Autodesk Inventor part; units mm, degrees
ref_plane "Work Plane1" through (0, -1.5, 0) normal (0, -1, 0) x (1, 0, 0)
ref_plane "YZ Plane" through (0, 0, 0) normal (1, 0, 0) x (0, 1, 0)
ref_plane "XZ Plane" through (0, 0, 0) normal (0, 1, 0) x (-1, 0, 0)
sketch "Sketch2" plane through (0, 0, 0) normal (0, 1, 0) x (-1, 0, 0)
  line L0 (-13.1182, 6.5103) -> (18.7692, 6.5103) construction
  line L1 (18.7692, 6.5103) -> (18.7692, -12.5367) construction
  line L2 (18.7692, -12.5367) -> (-13.1182, -12.5367) construction
  line L3 (-13.1182, -12.5367) -> (-13.1182, 6.5103) construction
  line L4 (-5.4, 3.15) -> (5.4, 3.15)
  line L5 (8.55, 0) -> (8.55, 0)
  line L6 (5.4, -3.15) -> (-5.4, -3.15)
  line L7 (-8.55, 0) -> (-8.55, 0)
  line L8 (-8.55, 3.15) -> (8.55, -3.15) construction
  line L9 (8.55, 3.15) -> (-8.55, -3.15) construction
  arc A0 (8.55, 0) -> (5.4, 3.15) centre (5.4, 0) ccw
  arc A1 (5.4, -3.15) -> (8.55, 0) centre (5.4, 0) ccw
  arc A2 (-5.4, 3.15) -> (-8.55, 0) centre (-5.4, 0) ccw
  arc A3 (-8.55, 0) -> (-5.4, -3.15) centre (-5.4, 0) ccw
  line L10 (5.4, 2.35) -> (-5.4, 2.35)
  line L11 (-7.75, 0) -> (-7.75, 0)
  line L12 (-5.4, -2.35) -> (5.4, -2.35)
  line L13 (7.75, 0) -> (7.75, 0)
  line L14 (7.75, 2.35) -> (-7.75, -2.35) construction
  line L15 (-7.75, 2.35) -> (7.75, -2.35) construction
  arc A4 (-5.4, 2.35) -> (-7.75, 0) centre (-5.4, 0) ccw
  arc A5 (-7.75, 0) -> (-5.4, -2.35) centre (-5.4, 0) ccw
  arc A6 (7.75, 0) -> (5.4, 2.35) centre (5.4, 0) ccw
  arc A7 (5.4, -2.35) -> (7.75, 0) centre (5.4, 0) ccw
  circle A8 centre (5.4, 0) radius 1.5
  circle A9 centre (-5.4, 0) radius 1.5
  circle A10 centre (2.3, 0) radius 0.9
  circle A11 centre (0, 0) radius 0.9
  circle A12 centre (-2.3, 0) radius 0.9
  circle A13 centre (2.3, 0) radius 0.35
  circle A14 centre (0, 0) radius 0.35
  circle A15 centre (-2.3, 0) radius 0.35
  point P0 (-7.75, 0)
  point P1 (7.75, 0)
  point P2 (-8.55, 0)
  point P3 (8.55, 0)
  dimension "d61" = 17.1
  dimension "d62" = 6.3
  dimension "d88" = 3.15
  dimension "d90" = 0.8
  dimension "d91" = 0.8
  dimension "d92" = 2.35
  dimension "d93" = 3
  dimension "d94" = 3
  dimension "d97" = 1.8
  dimension "d98" = 1.8
  dimension "d99" = 1.8
  dimension "d100" = 4.6
  dimension "d115" = 0.7
  dimension "d116" = 0.7
  dimension "d117" = 0.7
  dimension "d133" = 4.7
extrude "Extrusion1" add sketch "Sketch2" along normal blind 3.5 contours A6 A7 L12 A5 A4 L10 | A8 | A9 | A10 | A11 | A12 | A13 | A14 | A15
extrude "Extrusion2" add sketch "Sketch2" along normal blind 1.9 contours L4 A0 A1 L6 A3 A2
extrude "Extrusion3" cut sketch "Sketch2" along normal through all contours A10 | A11 | A12 | A13 | A14 | A15
ref_plane "Work Plane1" through (0, -1.5, 0) normal (0, -1, 0) x (1, 0, 0)
extrude "Extrusion5" add sketch "Sketch2" along normal blind 2 contours A10 | A11 | A12
sketch "Sketch5" plane through (0, 3.5, 0) normal (0, 1, 0) x (1, 0, 0)
  line L0 (0, 0) -> (5.4, 0)
  circle A0 centre (5.4, 0) radius 1.5
  line L1 (0, 0) -> (-5.4, 0)
  circle A1 centre (-5.4, 0) radius 1.5
  dimension "d127" = 5.4
  dimension "d128" = 3
  dimension "d129" = 5.4
  dimension "d130" = 3
extrude "Extrusion7" cut sketch "Sketch5" against normal blind 2
properties part number "Pogo1" material "Nylon 6"
For this review, take the finished solid that the model builds, in its own axes (mm). A direction names the side the tool comes from. Coordinates: 2 decimals unless noted, no trailing zeros. Write each loop counter-clockwise with the first axis right and the second up, starting at its lowest first coordinate (ties: lowest second). Pieces come first, ordered by that corner, then holes.
(1) Tool access review of faces 4 (the face through (0, 3, 2.35)), 5 (the face through (7.75, 2.69, -0.05)), 6 (the face through (-1.4, 2.7, 0)): name each direction out of +Z, -Z, +X, -X, +Y, -Y from which nothing blocks a thin tool from reaching the whole face with its end or side.
(2) Add section B-B on x = 0. Give the boundary of the cut face in (y, z), then the cut area to 3 significant figures.
(3) Add section A-A on y = 2.8. Give the boundary of the cut face in (x, z).
(4) The part is to be moulded in two halves that separate along X. For faces 1 (the face through (8.55, 0.94, -0.07)), 2 (the face through (3, 2, 0)), 3 (the face through (0, 1, 3.15)), say which applies: +X half, -X half, draft (parallel to the pull), parting line (faces both ways), or undercut.
(5) For pin 1 Ø0.5 at (x, z) = (0, -0.5) entering from +Y; pin 2 Ø1.3 at (x, y) = (1.5, 3) entering from +Z; pin 3 Ø1.5 at (x, z) = (5.5, 0) entering from +Y, all flat-tipped, find the tip position at first contact; note any pin that passes through.
(6) Wall thickness on probe 1 along X at (y, z) = (3.15, 0); probe 2 along Z at (x, y) = (0, 3.05); probe 3 along Z at (x, y) = (2.3, 0.8): over which ranges is each line inside the solid? List them lowest first.
(7) Add section C-C on y = 0.45. Give the boundary of the cut face in (x, z), then the cut area to 3 significant figures.
(8) Add section D-D on z = 0. Count the separate pieces of the cut face and the enclosed holes in it, then the cut area to 3 significant figures.
Answer sheet:
1. face 4: +Z, +X, -X, +Y
1. face 5: +X, +Y
1. face 6: +Y
2. outline: (0, -3.15) - (1.9, -3.15) - (1.9, -2.35) - (3.5, -2.35) - (3.5, -0.9) - (2, -0.9) - (2, -0.35) - (0, -0.35) - close; (0, 0.35) - (2, 0.35) - (2, 0.9) - (3.5, 0.9) - (3.5, 2.35) - (1.9, 2.35) - (1.9, 3.15) - (0, 3.15) - close
2. area: 15.4 mm2
3. outline: (-5.4, -2.35) - (5.4, -2.35) arc R2.35 ccw to (5.4, 2.35) - (-5.4, 2.35) arc R2.35 ccw to start; hole circle Ø3 at (-5.4, 0); hole circle Ø1.8 at (-2.3, 0); hole circle Ø1.8 at (0, 0); hole circle Ø1.8 at (2.3, 0); hole circle Ø3 at (5.4, 0)
4. face 1: +X half
4. face 2: undercut
4. face 3: draft
5. pin 1: stops at y = 2
5. pin 2: stops at z = 2.35
5. pin 3: stops at y = 1.5
6. probe 1: x = -7.75 to -6.9, -3.9 to -3.2, -1.4 to -0.9, 0.9 to 1.4, 3.2 to 3.9, 6.9 to 7.75
6. probe 2: z = -2.35 to -0.9, 0.9 to 2.35
6. probe 3: z = -3.15 to -0.35, 0.35 to 3.15
7. outline: (-5.4, -3.15) - (5.4, -3.15) arc R3.15 ccw to (5.4, 3.15) - (-5.4, 3.15) arc R3.15 ccw to start; hole circle Ø0.7 at (-2.3, 0); hole circle Ø0.7 at (0, 0); hole circle Ø0.7 at (2.3, 0)
7. area: 98.1 mm2
8. separate pieces: 4
8. enclosed holes: 0
8. area: 33.0 mm2
